Can you work these out from the model? Positions are in its coordinate system, mm. A direction names the side the tool comes from. Give positions to 0.01 mm unless a question says otherwise; leave off trailing zeros. Write each loop counter-clockwise with the first axis right and the second up, starting at its lowest first coordinate (ties: lowest second). Pieces come first, ordered by that corner, then holes.
Autodesk Inventor part; units mm, degrees
ref_plane "N_XY" through (-10, 0, 0) normal (-1, 0, 0) x (0, 0, -1)
ref_plane "N_YZ" through (-10, 0, 0) normal (0, 0, -1) x (0, -1, 0)
ref_plane "N_ZX" through (-10, 0, 0) normal (0, -1, 0) x (-1, 0, 0)
sketch "Sketch_1" plane through (0, 0, 0) normal (0, 0, 1) x (1, 0, 0)
  line L0 (99, 0) -> (-4, 0)
  line L1 (-4, 0) -> (-4, 2)
  line L2 (-4, 2) -> (71, 2)
  line L3 (71, 2) -> (71, 5)
  line L4 (71, 5) -> (99, 5)
  line L5 (99, 5) -> (99, 0)
  line L6 (99, 0) -> (-4, 0)
revolve "Revolution1" add sketch "Sketch_1" angle 360 about axis through (99, 0, 0) along (1, 0, 0)
sketch "Sketch_2" plane through (0, 0, 0) normal (0, 0, 1) x (1, 0, 0)
  line L0 (-4, 0) -> (-16, 0)
  line L1 (-16, 0) -> (-16, 1.5705)
  line L2 (-16, 1.5705) -> (-15.5705, 2)
  line L3 (-15.5705, 2) -> (-4.4295, 2)
  line L4 (-4.4295, 2) -> (-4, 1.5705)
  line L5 (-4, 1.5705) -> (-4, 0)
  line L6 (-4, 0) -> (-16, 0)
revolve "Revolution2" add sketch "Sketch_2" angle 360 about axis through (-4, 0, 0) along (1, 0, 0)
thread "Thread1"
ref_plane "N_XY" through (-10, 0, 0) normal (-1, 0, 0) x (0, 0, -1)
ref_plane "N_YZ" through (-10, 0, 0) normal (0, 0, -1) x (0, -1, 0)
ref_plane "N_ZX" through (-10, 0, 0) normal (0, -1, 0) x (-1, 0, 0)
ref_plane "N2_XY" through (174, 0, 0) normal (1, 0, 0) x (0, 0, -1)
ref_plane "N2_YZ" through (174, 0, 0) normal (0, 0, -1) x (0, 1, 0)
ref_plane "N2_ZX" through (174, 0, 0) normal (0, 1, 0) x (1, 0, 0)
ref_plane "P_XY" through (0, 0, 0) normal (1, 0, 0) x (0, 0, -1)
ref_plane "P_YZ" through (0, 0, 0) normal (0, 0, -1) x (0, 1, 0)
ref_plane "P_ZX" through (0, 0, 0) normal (0, 1, 0) x (1, 0, 0)
ref_plane "dim_am1_XY" through (-16, 1.5705, 0) normal (0, 0, 1) x (1, 0, 0)
ref_plane "dim_am1_YZ" through (-16, 1.5705, 0) normal (1, 0, 0) x (0, 1, 0)
ref_plane "dim_am1_ZX" through (-16, 1.5705, 0) normal (0, 1, 0) x (0, 0, 1)
ref_plane "dim_am2_XY" through (-4, 1.5705, 0) normal (0, 0, 1) x (1, 0, 0)
ref_plane "dim_am2_YZ" through (-4, 1.5705, 0) normal (1, 0, 0) x (0, 1, 0)
ref_plane "dim_am2_ZX" through (-4, 1.5705, 0) normal (0, 1, 0) x (0, 0, 1)
ref_plane "dim_bs1_XY" through (71, 5, 0) normal (0, 0, 1) x (1, 0, 0)
ref_plane "dim_bs1_YZ" through (71, 5, 0) normal (1, 0, 0) x (0, 1, 0)
ref_plane "dim_bs1_ZX" through (71, 5, 0) normal (0, 1, 0) x (0, 0, 1)
ref_plane "dim_bs2_XY" through (71, -5, 0) normal (0, 0, 1) x (1, 0, 0)
ref_plane "dim_bs2_YZ" through (71, -5, 0) normal (1, 0, 0) x (0, 1, 0)
ref_plane "dim_bs2_ZX" through (71, -5, 0) normal (0, 1, 0) x (0, 0, 1)
ref_plane "dim_mm1_XY" through (-4, 2, 0) normal (0, 0, 1) x (1, 0, 0)
ref_plane "dim_mm1_YZ" through (-4, 2, 0) normal (1, 0, 0) x (0, 1, 0)
ref_plane "dim_mm1_ZX" through (-4, 2, 0) normal (0, 1, 0) x (0, 0, 1)
ref_plane "dim_mm2_XY" through (-4, -2, 0) normal (0, 0, 1) x (1, 0, 0)
ref_plane "dim_mm2_YZ" through (-4, -2, 0) normal (1, 0, 0) x (0, 1, 0)
ref_plane "dim_mm2_ZX" through (-4, -2, 0) normal (0, 1, 0) x (0, 0, 1)
properties part number "RM/8010/M/50_0_0_P"
1) Suppose I cut it at A-A on y = 0. Write out the boundary of the cut face in (x, z).
Values follow:
outline: (-16, -1.57) - (-15.57, -2) - (-4.43, -2) - (-4, -1.57) - (-4, -2) - (71, -2) - (71, -5) - (99, -5) - (99, 5) - (71, 5) - (71, 2) - (-4, 2) - (-4, 1.57) - (-4.43, 2) - (-15.57, 2) - (-16, 1.57) - close
2) For pin 1 Ø1.5 at (x, y) = (-4, 1.5) entering from -Z; pin 2 Ø5 at (x, y) = (54, -0.5) entering from +Z; pin 3 Ø6 at (x, y) = (27, -1) entering from -Z; pin 4 Ø1.5 at (x, y) = (6, -3.5) entering from +Z, each with a flat end and sliding along its axis, tell me the tip position at first contact or that it passes through.
Values follow:
pin 1: stops at z = -1.85
pin 2: stops at z = 2
pin 3: stops at z = -2
pin 4: passes through
3) Suppose I cut it at C-C on x = 0. Write out the boundary of the cut face in (y, z), plus the area to 3 significant figures.
Values follow:
outline: circle Ø4 at (0, 0)
area: 12.6 mm2
4) Please list where these lines run through material, in increasing order: L1, parallel to X at y = -2, z = -1; L2, parallel to X at y = -1.5, z = 1.25; L3, parallel to Z at x = 54, y = -1.25.
Values follow:
L1: x = 71 to 99
L2: x = -15.62 to -4.38, -4 to 99
L3: z = -1.56 to 1.56
5) For faces 1 (the face through (-10, 0, -2)), 2 (the face through (-16, 0, 0)), which set-ups out of +Z, -Z, +X, -X, +Y, -Y let a thin tool reach every point of the face, with its end or its side?
Values follow:
face 1: -X
face 2: +Z, -Z, -X, +Y, -Y
